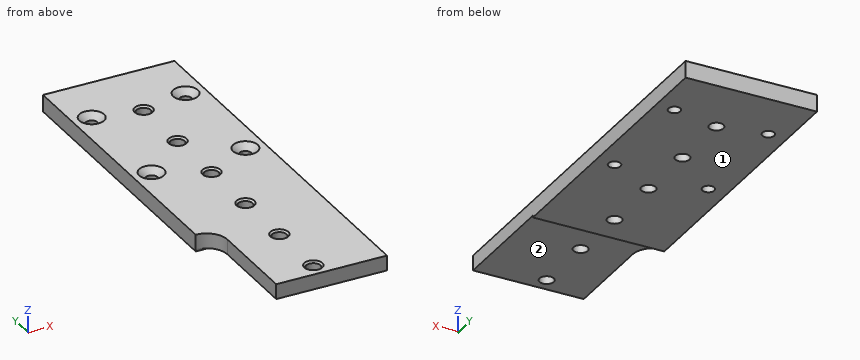
Autodesk Inventor part; units mm, degrees
ref_plane "Work Plane1" through (-129, 13.9597, 0) normal (1, 0, 0) x (0, 1, 0)
ref_plane "YZ Plane" through (0, 0, 0) normal (1, 0, 0) x (0, 1, 0)
ref_plane "XZ Plane" through (0, 0, 0) normal (0, 1, 0) x (-1, 0, 0)
sketch "Sketch1" plane through (0, 0, 0) normal (0, 0, 1) x (1, 0, 0)
  line L0 (-146.5, 49) -> (-146.5, 125.5)
  line L1 (-146.5, 125.5) -> (-111.5, 125.5)
  line L2 (-111.5, 125.5) -> (-111.5, 19)
  line L3 (-111.5, 19) -> (-141, 19)
  line L4 (-141, 19) -> (-141, 43.5)
  arc A0 (-141, 43.5) -> (-146.5, 49) centre (-146.5, 43.5) ccw
  line L5 (-129, 13.9597) -> (-129, 176.9597)
  circle A1 centre (-129, 23) radius 1.9
  circle A2 centre (-129, 40) radius 1.9
  circle A3 centre (-129, 57) radius 1.9
  circle A4 centre (-129, 74) radius 1.9
  circle A5 centre (-129, 91) radius 1.9
  circle A6 centre (-129, 108) radius 1.9
  circle A7 centre (-141.5, 80.5) radius 3.3
  circle A8 centre (-141.5, 80.5) radius 1.6
  line L6 (-154.2414, 80.5) -> (-103.7586, 80.5) construction
  circle A9 centre (-141.5, 110.5) radius 1.6
  circle A10 centre (-141.5, 110.5) radius 3.3
  circle A11 centre (-116.5, 80.5) radius 3.3
  circle A12 centre (-116.5, 80.5) radius 1.6
  circle A13 centre (-116.5, 110.5) radius 1.6
  circle A14 centre (-116.5, 110.5) radius 3.3
  line L7 (-146.5, 49) -> (-111.5, 49)
  point P0 (0, 0)
  dimension "d0" = 5.5
  dimension "d1" = 76.5
  dimension "d2" = 35
  dimension "d3" = 106.5
  dimension "d5" = 17.5
  dimension "d6" = 3.8
  dimension "d9" = 17
  dimension "d14" = 85
  dimension "d15" = 4
  dimension "d16" = 6.6
  dimension "d17" = 3.2
  dimension "d20" = 30
  dimension "d25" = 30
  dimension "d53" = 5
  dimension "d54" = 15
extrude "Extrusion1" add sketch "Sketch1" against normal blind 4.5 contours L0 L1 L5 A6 A5 A4 A3 L7 | L5 A3 A4 A5 A6 L1 L2 L7 | A7 | A10 | A11 | A14
sketch "Sketch2" plane through (0, 0, 0) normal (0, 0, 1) x (1, 0, 0)
  circle A0 centre (-141.5, 80.5) radius 1.6
  circle A1 centre (-141.5, 110.5) radius 1.6
  circle A2 centre (-116.5, 110.5) radius 1.6
  circle A3 centre (-116.5, 80.5) radius 1.6
  point P0 (0, 0)
hole "Hole1" at (-141.5, 80.5, 0) at (-141.5, 110.5, 0) at (-116.5, 110.5, 0) at (-116.5, 80.5, 0) direction (0, 0, -1) diameter 3.2 end through all countersink diameter 6.6 countersink angle 90
extrude "Extrusion2" add sketch "Sketch1" against normal blind 4 contours L7 L5 A2 A1 L3 L4 A0 | L7 L2 L3 L5 A1 A2
chamfer "Chamfer1" distance 0.5 angle 45 6 edges at (-130.9, 108, 0) (-130.9, 91, 0) (-130.9, 74, 0) (-130.9, 57, 0) (-130.9, 40, 0) (-130.9, 23, 0) measured on face at (-117.6556, 51.1917, 0)
thread "Thread1"
thread "Thread2"
thread "Thread3"
thread "Thread4"
thread "Thread5"
thread "Thread6"
ref_plane "Work Plane1" through (-129, 13.9597, 0) normal (1, 0, 0) x (0, 1, 0)
equation "\"d6\" = m4"
equation "\"m3\" = 2.8"
equation "\"m4\" = 3.8"
properties part number "АНЦП.014.00.00.005" material "PET Plastic"
Can you work these out from the model? Positions are in its coordinate system, mm. Face numbers are marked on the shaded views. A direction names the side the tool comes from. Coordinates: 2 decimals unless noted, no trailing zeros. Order: outer loops, then holes, each group sorted by start corner. A loop starts at its lowest first (then second) coordinate and runs counter-clockwise, first axis right, second up. Notation, with made-up numbers: (-9, 75.5) - (16, 75.5) arc R17 ccw to (16, 82.5) - close; hole circle Ø11 at (78.5, 47). An arc over 180 degrees is marked (long way). Answer in a Markdown table with one row per item.
1. Suppose I cut it at C-C (y = 80.5). Please give me the cut outline in (x, z).
Reply:
| item | result |
|---|---|
| outline | (-146.5, -4.5) - (-143.1, -4.5) - (-143.1, -1.7) - (-144.8, 0) - (-146.5, 0) - close; (-139.9, -4.5) - (-118.1, -4.5) - (-118.1, -1.7) - (-119.8, 0) - (-138.2, 0) - (-139.9, -1.7) - close; (-114.9, -4.5) - (-111.5, -4.5) - (-111.5, 0) - (-113.2, 0) - (-114.9, -1.7) - close |
2. If I drill on line 1 along X through (y, z) = (110.5, -2.85); line 2 along Y through (x, z) = (-116.5, -3.55); line 3 along X through (y, z) = (108, -2.25), over which ranges is the centre line in solid material (lowest first)?
Reply:
| item | result |
|---|---|
| line 1 | x = -146.5 to -143.1, -139.9 to -118.1, -114.9 to -111.5 |
| line 2 | y = 19 to 78.9, 82.1 to 108.9, 112.1 to 125.5 |
| line 3 | x = -146.5 to -130.9, -127.1 to -111.5 |
3. For pin 1 (4.5 mm diameter, centred on x = -129, y = 40, fed in from -Z), with a flat end and sliding along its axis, tell me the tip position at first contact or that it passes through.
Reply:
| item | result |
|---|---|
| pin 1 | stops at z = -4 |
4. Suppose I cut it at A-A (y = 40). Please give me the cut outline in (x, z), and give its area (3 significant figures).
Reply:
| item | result |
|---|---|
| outline | (-141, -4) - (-130.9, -4) - (-130.9, -0.5) - (-131.4, 0) - (-141, 0) - close; (-127.1, -4) - (-111.5, -4) - (-111.5, 0) - (-126.6, 0) - (-127.1, -0.5) - close |
| area | 103 mm^2 |
5. For the marked faces 1 and 2, which set-ups out of +Z, -Z, +X, -X, +Y, -Y let a thin tool reach every point of the face, with its end or its side?
Reply:
| item | result |
|---|---|
| face 1 | -Z, +X, -X, +Y, -Y |
| face 2 | -Z, +X, -X, -Y |
6. Suppose I cut it at D-D (x = -129). Give the number of separate pieces and of enclosed holes in the cut face, and give its area (3 significant figures).
Reply:
| item | result |
|---|---|
| separate pieces | 7 |
| enclosed holes | 0 |
| area | 364 mm^2 |
7. Suppose I cut it at B-B (x = -116.5). Please give me the cut outline in (y, z), and give its area (3 significant figures).
Reply:
| item | result |
|---|---|
| outline | (19, -4) - (49, -4) - (49, -4.5) - (78.9, -4.5) - (78.9, -1.7) - (77.2, 0) - (19, 0) - close; (82.1, -4.5) - (108.9, -4.5) - (108.9, -1.7) - (107.2, 0) - (83.8, 0) - (82.1, -1.7) - close; (112.1, -4.5) - (125.5, -4.5) - (125.5, 0) - (113.8, 0) - (112.1, -1.7) - close |
| area | 430 mm^2 |
